Here's the drawing with two shaded views (mm, measured from the low corner). I have some questions. A direction names the side the tool comes from. Coordinates: 2 decimals unless noted, no trailing zeros. Write each loop counter-clockwise with the first axis right and the second up, starting at its lowest first coordinate (ties: lowest second). Pieces come first, ordered by that corner, then holes.
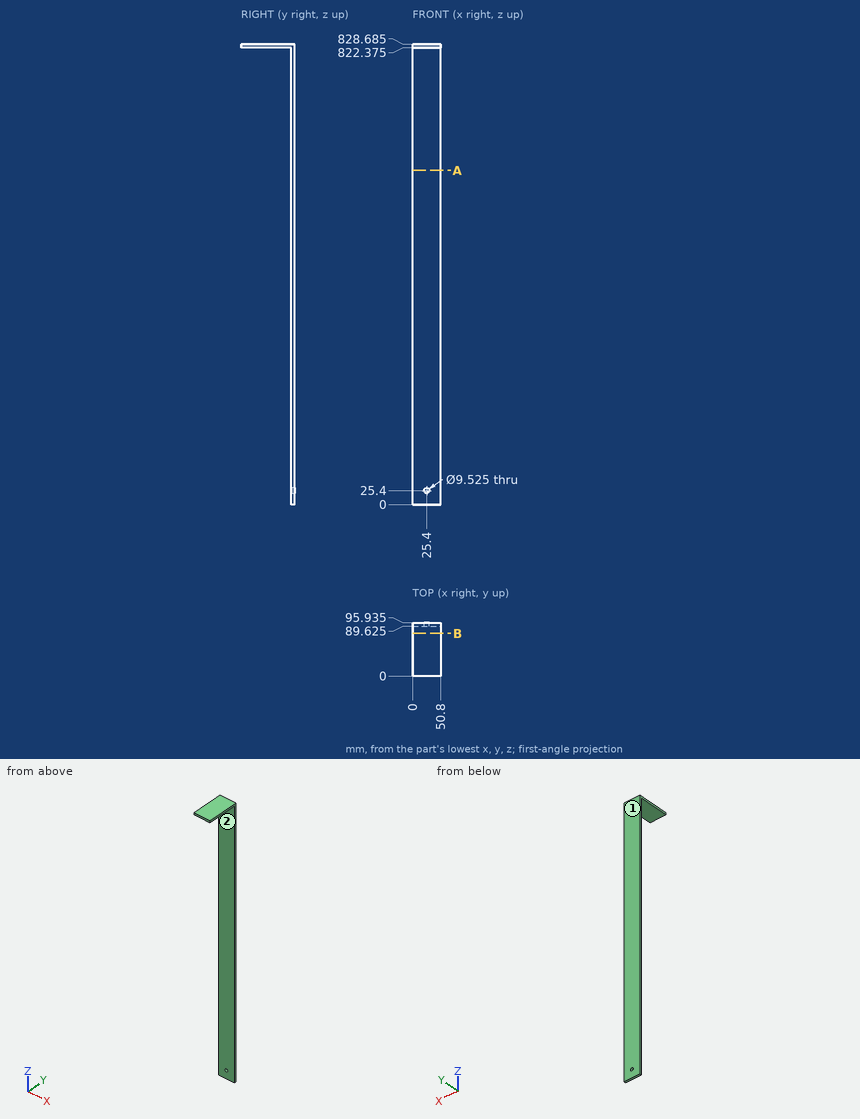
1. On a 3-axis mill with a long thin cutter (end or side, diameter ignored), from which of +Z, -Z, +X, -X, +Y, -Y can I reach the whole of each face in a straight line? I mean the marked faces 1 and 2. Say none if no direction works.
Verdict:
face 1: +Z, -Z, +X, -X, +Y
face 2: -Z, +X, -X, -Y
2. I want a section at B-B on y = 76.5. Please give me the cut outline in (x, z) (3 decimals).
Verdict:
outline: (0, 822.375) - (50.8, 822.375) - (50.8, 828.685) - (0, 828.685) - close
3. I want a section at A-A on z = 601.5. Please give me the cut outline in (x, y) (3 decimals), plus the area to 3 significant figures.
Verdict:
outline: (0, 89.625) - (50.8, 89.625) - (50.8, 95.935) - (0, 95.935) - close
area: 321 mm2
4. Please list where these lines run through material, in increasing order: line 1 along X through (y, z) = (91.5, 25.4); line 2 along Z through (x, y) = (25, 92) (3 decimals); line 3 along X through (y, z) = (91, 25).
Verdict:
line 1: x = 0 to 20.64, 30.16 to 50.8
line 2: z = 0 to 20.654, 30.146 to 828.685
line 3: x = 0 to 20.65, 30.15 to 50.8
5. For pin 1 (6 mm diameter, centred on x = 12, z = 290, fed in from -Y) (3 decimals); pin 2 (15 mm diameter, centred on x = 37.5, y = 56, fed in from -Z) (3 decimals), each with a flat end and sliding along its axis, tell me the tip position at first contact or that it passes through.
Verdict:
pin 1: stops at y = 89.625
pin 2: stops at z = 822.375
